```python
from build123d import *

# Parameters (mm, degrees)
SKETCH1_W                      = 45
SKETCH1_H                      = 45
SKETCH1_R                      = 16
BOSS_EXTRUDE1_DEPTH            = 7.1
M3X0_5_TAPPED_HOLE1_D          = 2.5
M3X0_5_TAPPED_HOLE1_DEPTH      = 15
M3X0_5_TAPPED_HOLE1_TIP        = 0.751075774
CBORE_FOR_M3_SHCS1_D           = 3.4
CBORE_FOR_M3_SHCS1_DEPTH       = 7.1
CBORE_FOR_M3_SHCS1_CBORE_D     = 6.5
CBORE_FOR_M3_SHCS1_CBORE_DEPTH = 3
CBORE_FOR_M3_SHCS1_TIP         = 1.021463052
F_3D_PRINTING_TOLERANCE_BY     = 0.05


with BuildPart() as part:
    # Sketch1 → Boss-Extrude1 (new body)
    with BuildSketch(Plane.XY):
        Rectangle(SKETCH1_W, SKETCH1_H)
        Circle(SKETCH1_R, mode=Mode.SUBTRACT)
    extrude(amount=BOSS_EXTRUDE1_DEPTH)

    # M3x0.5 Tapped Hole1
    with Locations(Plane(origin=(0, 0, 0), x_dir=(-1, 0, 0), z_dir=(0, 0, -1))):
        with Locations((-18.5, 18.5), (-18.5, -18.5), (18.5, -18.5), (18.5, 18.5)):
            Hole(M3X0_5_TAPPED_HOLE1_D / 2, depth=M3X0_5_TAPPED_HOLE1_DEPTH)
            with Locations((0, 0, -(M3X0_5_TAPPED_HOLE1_DEPTH + M3X0_5_TAPPED_HOLE1_TIP / 2))):  # 118° drill point
                Cone(0, M3X0_5_TAPPED_HOLE1_D / 2, M3X0_5_TAPPED_HOLE1_TIP, mode=Mode.SUBTRACT)

    # CBORE for M3 SHCS1
    with Locations(Plane(origin=(0, 0, 0), x_dir=(-1, 0, 0), z_dir=(0, 0, -1))):
        with Locations((-18.5, 18.5), (18.5, 18.5), (18.5, -18.5), (-18.5, -18.5)):
            CounterBoreHole(CBORE_FOR_M3_SHCS1_D / 2, CBORE_FOR_M3_SHCS1_CBORE_D / 2, CBORE_FOR_M3_SHCS1_CBORE_DEPTH, depth=CBORE_FOR_M3_SHCS1_DEPTH)
            with Locations((0, 0, -(CBORE_FOR_M3_SHCS1_DEPTH + CBORE_FOR_M3_SHCS1_TIP / 2))):  # 118° drill point
                Cone(0, CBORE_FOR_M3_SHCS1_D / 2, CBORE_FOR_M3_SHCS1_TIP, mode=Mode.SUBTRACT)

    # 3D Printing Tolerance: a curved face moved inward by 0.05
    add(Solid.thicken(part.faces().sort_by_distance((-16, 0, 3.55))[0], -F_3D_PRINTING_TOLERANCE_BY), mode=Mode.SUBTRACT)


solid = part.part
```
Geometry check sheet. Reference: the model listing, model coordinates, mm. A direction names the side the tool comes from. Round coordinates to 2 decimals unless told otherwise and drop trailing zeros. Loops run counter-clockwise (first coordinate to the right, second up) from the corner with the lowest first, then second, coordinate; pieces in that order, holes last. Notation, with made-up numbers: (34, -6.5) - (80, -6.5) arc R23 ccw to (80, 5.5) - close; hole circle Ø7 at (-22, 88.25). An arc over 180 degrees is marked (long way). Write item = value, one per line. Start each with the question number.
1. Thickness scan on line 1 (X direction, y = 18.5, z = 4.7); line 2 (Y direction, x = -18.5, z = 1.95). Record the ranges inside material, lowest first.
2. Section check A-A on x = 0. Enter the section's corners in (y, z).
3. Depth check by flat-ended pin: pin 1 (3 mm diameter, centred on x = -18.5, y = -18.5, fed in from +Z); pin 2 (8 mm diameter, centred on x = 9, y = 13, fed in from +Z); pin 3 (4 mm diameter, centred on x = -18.5, y = -18.5, fed in from -Z). Enter the tip coordinate at first touch or a pass-through.
4. Section check D-D on y = -18.5. Enter the section's corners in (x, z).
5. Section check C-C on z = 2. Enter the section's corners in (x, y), then the cut area to 3 significant figures.
6. Set-up check for faces 1 (the face through (19.414, 19.933, 5.079)), 2 (the face through (21.747, 18.643, 1.479)): record each of +Z, -Z, +X, -X, +Y, -Y from which the full face is reachable in a straight line by a thin tool's end or side.
Working result:
q1.line_1 = -22.5 to -20.2, -16.8 to 16.8, 20.2 to 22.5
q1.line_2 = -22.5 to -21.75, -15.25 to 15.25, 21.75 to 22.5
q2.outline = (-22.5, 0) - (-16.05, 0) - (-16.05, 7.1) - (-22.5, 7.1) - close; (16.05, 0) - (22.5, 0) - (22.5, 7.1) - (16.05, 7.1) - close
q3.pin_1 = through
q3.pin_2 = 7.1
q3.pin_3 = 3
q4.outline = (-22.5, 0) - (-21.75, 0) - (-21.75, 3) - (-20.2, 3) - (-20.2, 7.1) - (-22.5, 7.1) - close; (-16.8, 3) - (-15.25, 3) - (-15.25, 0) - (15.25, 0) - (15.25, 3) - (16.8, 3) - (16.8, 7.1) - (-16.8, 7.1) - close; (20.2, 3) - (21.75, 3) - (21.75, 0) - (22.5, 0) - (22.5, 7.1) - (20.2, 7.1) - close
q5.outline = (-22.5, -22.5) - (22.5, -22.5) - (22.5, 22.5) - (-22.5, 22.5) - close; hole circle Ø6.5 at (-18.5, -18.5); hole circle Ø6.5 at (-18.5, 18.5); hole circle Ø32.1 at (0, 0); hole circle Ø6.5 at (18.5, -18.5); hole circle Ø6.5 at (18.5, 18.5)
q5.area = 1,080 mm^2
q6.face_1 = +Z, -Z
q6.face_2 = -Z
